```python
from build123d import *

# Parameters (mm, degrees)
SKETCH1_R           = 1.5
BOSS_EXTRUDE2_DEPTH = 6
SKETCH2_R           = 1.5
SKETCH2_R_2         = 2
SKETCH2_R_3         = 11.5
CUT_EXTRUDE1_DEPTH  = 6
BOSS_EXTRUDE3_DEPTH = 6
CHAMFER1_SIZE       = 15
FILLET1_R           = 5


with BuildPart() as part:
    # Sketch1 → Boss-Extrude2 (new body)
    with BuildSketch(Plane(origin=(0, 0, 0), x_dir=(1, 0, 0), z_dir=(0, 1, 0))):
        with BuildLine():
            Line((-46.904157598, -105), (46.904157598, -105))
            ThreePointArc((46.904157598, -105), (115, 0), (46.904157598, 105))
            Line((46.904157598, 105), (-46.904157598, 105))
            ThreePointArc((-46.904157598, 105), (-115, 0), (-46.904157598, -105))
        make_face()
        with Locations((-30, 100)):
            Circle(SKETCH1_R, mode=Mode.SUBTRACT)
        with Locations((30, 100)):
            Circle(SKETCH1_R, mode=Mode.SUBTRACT)
        with Locations((30, 89)):
            Circle(SKETCH1_R, mode=Mode.SUBTRACT)
        with Locations((-30, 89)):
            Circle(SKETCH1_R, mode=Mode.SUBTRACT)
        with Locations((-30, -89)):
            Circle(SKETCH1_R, mode=Mode.SUBTRACT)
        with Locations((30, -89)):
            Circle(SKETCH1_R, mode=Mode.SUBTRACT)
        with Locations((30, -100)):
            Circle(SKETCH1_R, mode=Mode.SUBTRACT)
        with Locations((-30, -100)):
            Circle(SKETCH1_R, mode=Mode.SUBTRACT)
    extrude(amount=BOSS_EXTRUDE2_DEPTH)

    # Sketch2 → Cut-Extrude1 (cut)
    with BuildSketch(Plane(origin=(0, 6, 0), x_dir=(1, 0, 0), z_dir=(0, 1, 0))):
        with Locations((-50, 22)):
            Circle(SKETCH2_R)
        with Locations((-19, 22)):
            Circle(SKETCH2_R)
        with Locations((-19, -20)):
            Circle(SKETCH2_R)
        with Locations((-50, -20)):
            Circle(SKETCH2_R)
        with Locations((80, 40)):
            Circle(SKETCH2_R)
        with Locations((30.47, 40)):
            Circle(SKETCH2_R)
        with Locations((30.47, -20.96)):
            Circle(SKETCH2_R)
        with Locations((80, -20.96)):
            Circle(SKETCH2_R)
        with Locations((70, 80)):
            Circle(SKETCH2_R_2)
        with Locations((-70, 80)):
            Circle(SKETCH2_R_2)
        with Locations((-70, -80)):
            Circle(SKETCH2_R_2)
        with Locations((70, -80)):
            Circle(SKETCH2_R_2)
        with Locations((-100, 20)):
            Circle(SKETCH2_R_2)
        with Locations((-100, -20)):
            Circle(SKETCH2_R_2)
        with Locations((100, 20)):
            Circle(SKETCH2_R_2)
        with Locations((100, -20)):
            Circle(SKETCH2_R_2)
        with Locations((-100, 0)):
            Circle(SKETCH2_R_3)
        with Locations((100, 0)):
            Circle(SKETCH2_R_3)
    extrude(amount=-CUT_EXTRUDE1_DEPTH, mode=Mode.SUBTRACT)

    # Sketch4 → Boss-Extrude3 (add)
    with BuildSketch(Plane(origin=(0, 6, 0), x_dir=(1, 0, 0), z_dir=(0, 1, 0))):
        with BuildLine():
            ThreePointArc((-115, 0), (-96.485693561, 62.574043645), (-46.904157598, 105))
            Line((-46.904157598, 105), (-115, 105))
            Line((-115, 105), (-115, 0))
        make_face()
        with BuildLine():
            ThreePointArc((-46.904157598, -105), (-96.485693561, -62.574043645), (-115, 0))
            Line((-115, 0), (-115, -105))
            Line((-115, -105), (-46.904157598, -105))
        make_face()
    extrude(amount=-BOSS_EXTRUDE3_DEPTH)

    # Chamfer1
    chamfer1_edges = [part.edges().sort_by_distance(p)[0] for p in [
        (-115, 3, -105),
        (-115, 3, 105),
    ]]
    chamfer(chamfer1_edges, length=CHAMFER1_SIZE)

    # Fillet1
    fillet1_edges = [part.edges().sort_by_distance(p)[0] for p in [
        (-115, 3, -90),
        (-115, 3, 90),
        (-100, 3, 105),
        (-100, 3, -105),
    ]]
    fillet(fillet1_edges, radius=FILLET1_R)


solid = part.part
```
Part model, mm, in its own coordinate system. Give positions to 0.01 mm unless a question says otherwise; leave off trailing zeros. Write each loop counter-clockwise with the first axis right and the second up, starting at its lowest first coordinate (ties: lowest second). Pieces come first, ordered by that corner, then holes. Notation, with made-up numbers: M 78.25,42 L 94.25,42 A7 cw 94.25,52 Z; hole C 24,72.25 d2. An arc over 180 degrees is marked long. Use CSV: the item, a comma, the result in double quotes.
Item 1: Drill centre lines: probe 1 along Z at (x, y) = (-19, 2); probe 2 along Z at (x, y) = (-30, 3.95); probe 3 along X at (y, z) = (2.55, -20). Where is each one in solid material? Low to high.
Taken from the geometry:
probe 1,"z = -105 to -23.5, -20.5 to 18.5, 21.5 to 105"
probe 2,"z = -105 to -101.5, -98.5 to -90.5, -87.5 to 87.5, 90.5 to 98.5, 101.5 to 105"
probe 3,"x = -115 to -102, -98 to 98, 102 to 113.25"
Item 2: Slice it at C-C on x = 75. Write the cut outline in (y, z).
Taken from the geometry:
outline,"M 0,-87.18 L 6,-87.18 L 6,87.18 L 0,87.18 Z"
Item 3: Pull direction X, two halves, no side cores. Call faces 1 (the face through (-108.48, 3.04, -7.77)), 2 (the face through (-108, 3, -97)), 3 (the face through (-2, 6, -1)): +X half, -X half, draft (parallel to the pull), parting line (faces both ways), or undercut.
Taken from the geometry:
face 1,"undercut"
face 2,"-X half"
face 3,"draft"
Item 4: Slice it at B-B on z = 40. Write the cut outline in (x, y), plus the area to 3 significant figures.
Taken from the geometry:
outline,"M -115,0 L 107.82,0 L 107.82,6 L -115,6 Z"
area,"1,340 mm²"
Item 5: Slice it at A-A on y = 3.3. State how many separate pieces and enclosed holes the cut face has, plus the area to 3 significant figures.
Taken from the geometry:
separate pieces,"1"
enclosed holes,"26"
area,"43,000 mm²"
Item 6: Pin check, flat tip, straight feed: P1, Ø2.5, axis at x = -30, z = -89, coming from the -Y side. Stop position of the tip, or through.
Taken from the geometry:
P1,"passes through"
